Read the model definition and answer for the solid it produces. Units are mm, in the model's axes. Face numbers are marked on the shaded views. Coordinates: 2 decimals unless noted, no trailing zeros. Loops run counter-clockwise (first coordinate to the right, second up) from the corner with the lowest first, then second, coordinate; pieces in that order, holes last.
from build123d import *

# Parameters (mm, degrees)
SKETCH1_W           = 350
SKETCH1_H           = 56.2
BOSS_EXTRUDE1_DEPTH = 10
SKETCH2_W           = 56.2
SKETCH2_H           = 56.2
CUT_EXTRUDE1_DEPTH  = 5
SKETCH3_W           = 10
SKETCH3_H           = 56.2
BOSS_EXTRUDE2_DEPTH = 10
SKETCH4_W           = 10
SKETCH4_H           = 56.2
BOSS_EXTRUDE3_DEPTH = 10
CUT_EXTRUDE2_DEPTH  = 56.2
SKETCH6_W           = 10
SKETCH6_H           = 56.2
BOSS_EXTRUDE4_DEPTH = 10
SKETCH7_W           = 10
SKETCH7_H           = 56.2
BOSS_EXTRUDE5_DEPTH = 10
CUT_EXTRUDE3_DEPTH  = 56.2
SKETCH9_W           = 30
SKETCH9_H           = 30
CUT_EXTRUDE4_DEPTH  = 5
SKETCH10_R          = 3
CUT_EXTRUDE5_DEPTH  = 5
SKETCH11_W          = 2.5
SKETCH11_H          = 15
CUT_EXTRUDE6_DEPTH  = 7
SKETCH12_W          = 2.5
SKETCH12_H          = 15
CUT_EXTRUDE7_DEPTH  = 7
SKETCH13_W          = 100.7
SKETCH13_H          = 56.2
CUT_EXTRUDE9_DEPTH  = 10


with BuildPart() as part:
    # Sketch1 → Boss-Extrude1 (new body)
    with BuildSketch(Plane.XY):
        Rectangle(SKETCH1_W, SKETCH1_H)
    extrude(amount=BOSS_EXTRUDE1_DEPTH)

    # Sketch2 → Cut-Extrude1 (cut)
    with BuildSketch(Plane.XY.offset(10)):
        Rectangle(SKETCH2_W, SKETCH2_H)
    extrude(amount=-CUT_EXTRUDE1_DEPTH, mode=Mode.SUBTRACT)

    # Sketch3 → Boss-Extrude2 (add)
    with BuildSketch(Plane(origin=(175, 0, 0), x_dir=(0, 0, -1), z_dir=(1, 0, 0))):
        with Locations((-5, 0)):
            Rectangle(SKETCH3_W, SKETCH3_H)
    extrude(amount=BOSS_EXTRUDE2_DEPTH)

    # Sketch4 → Boss-Extrude3 (add)
    with BuildSketch(Plane.XY.offset(10)):
        with Locations((180, 0)):
            Rectangle(SKETCH4_W, SKETCH4_H)
    extrude(amount=BOSS_EXTRUDE3_DEPTH)

    # Sketch5 → Cut-Extrude2 (cut)
    with BuildSketch(Plane(origin=(0, 28.1, 0), x_dir=(1, 0, 0), z_dir=(0, 1, 0))):
        Polygon((175, -20), (185, -10), (185, -20), align=None)
    extrude(amount=-CUT_EXTRUDE2_DEPTH, mode=Mode.SUBTRACT)

    # Sketch6 → Boss-Extrude4 (add)
    with BuildSketch(Plane.ZY.offset(175)):
        with Locations((5, 0)):
            Rectangle(SKETCH6_W, SKETCH6_H)
    extrude(amount=BOSS_EXTRUDE4_DEPTH)

    # Sketch7 → Boss-Extrude5 (add)
    with BuildSketch(Plane.XY.offset(10)):
        with Locations((-180, 0)):
            Rectangle(SKETCH7_W, SKETCH7_H)
    extrude(amount=BOSS_EXTRUDE5_DEPTH)

    # Sketch8 → Cut-Extrude3 (cut)
    with BuildSketch(Plane(origin=(0, 28.1, 0), x_dir=(1, 0, 0), z_dir=(0, 1, 0))):
        Polygon((-175, -20), (-185, -10), (-185, -20), align=None)
    extrude(amount=-CUT_EXTRUDE3_DEPTH, mode=Mode.SUBTRACT)

    # Sketch9 → Cut-Extrude4 (cut)
    with BuildSketch(Plane.XY.offset(5)):
        Rectangle(SKETCH9_W, SKETCH9_H)
    extrude(amount=-CUT_EXTRUDE4_DEPTH, mode=Mode.SUBTRACT)

    # Sketch10 → Cut-Extrude5 (cut)
    with BuildSketch(Plane.XY.offset(5)):
        with Locations((21.55, 21.55)):
            Circle(SKETCH10_R)
        with Locations((-21.55, -21.55)):
            Circle(SKETCH10_R)
        with Locations((-21.55, 21.55)):
            Circle(SKETCH10_R)
        with Locations((21.55, -21.55)):
            Circle(SKETCH10_R)
    extrude(amount=-CUT_EXTRUDE5_DEPTH, mode=Mode.SUBTRACT)

    # Sketch11 → Cut-Extrude6 (cut)
    with BuildSketch(Plane(origin=(97.5, 0, 97.5), x_dir=(0.7071067811865478, 0, -0.7071067811865472), z_dir=(0.7071067811865472, 0, 0.7071067811865478))):
        with Locations((116.672618896, 0)):
            Rectangle(SKETCH11_W, SKETCH11_H)
    extrude(amount=-CUT_EXTRUDE6_DEPTH, mode=Mode.SUBTRACT)

    # Sketch12 → Cut-Extrude7 (cut)
    with BuildSketch(Plane(origin=(-97.5, 0, 97.5), x_dir=(0.7071067811865478, 0, 0.7071067811865472), z_dir=(-0.7071067811865472, 0, 0.7071067811865478))):
        with Locations((-116.672618896, 0)):
            Rectangle(SKETCH12_W, SKETCH12_H)
    extrude(amount=-CUT_EXTRUDE7_DEPTH, mode=Mode.SUBTRACT)

    # Sketch13 → Cut-Extrude9 (cut)
    with BuildSketch(Plane.XY.offset(10)):
        with Locations((-134.65, 0)):
            Rectangle(SKETCH13_W, SKETCH13_H)
        with Locations((134.65, 0)):
            Rectangle(SKETCH13_W, SKETCH13_H)
    extrude(amount=-CUT_EXTRUDE9_DEPTH, mode=Mode.SUBTRACT)


with BuildPart() as body_2:
    # of the pieces the cut leaves, the one that is kept (cut_extrude9_keep)
    add(part.part.solids().sort_by_distance((-84.3, -28.1, 0))[0])


solid = body_2.part
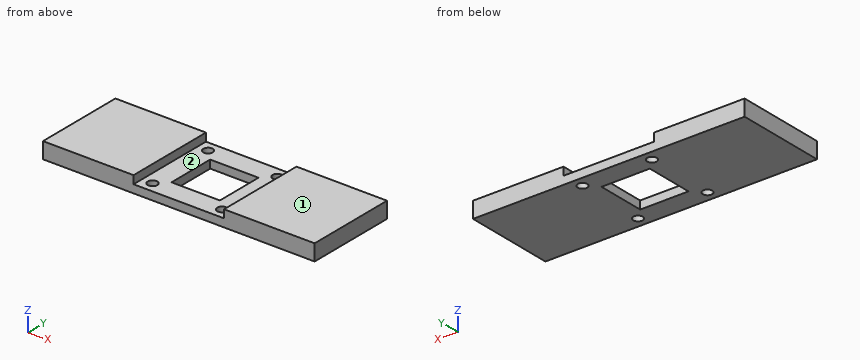
Item 1: A cutting plane is placed at A-A on z = 6.75. Determine the outline of the cut face in (x, y), then the cut area to 3 significant figures.
Numbers:
outline: (-84.3, -28.1) - (-28.1, -28.1) - (-28.1, 28.1) - (-84.3, 28.1) - close; (28.1, -28.1) - (84.3, -28.1) - (84.3, 28.1) - (28.1, 28.1) - close
area: 6,320 mm2
Item 2: A cutting plane is placed at B-B on x = -21.55. Determine the outline of the cut face in (y, z).
Numbers:
outline: (-28.1, 0) - (-24.55, 0) - (-24.55, 5) - (-28.1, 5) - close; (-18.55, 0) - (18.55, 0) - (18.55, 5) - (-18.55, 5) - close; (24.55, 0) - (28.1, 0) - (28.1, 5) - (24.55, 5) - close
Item 3: Given pin 1 (5 mm diameter, centred on x = -21.55, y = 21.55, fed in from +Z); pin 2 (9.5 mm diameter, centred on x = -21.55, y = -21.55, fed in from +Z), each flat-ended and moving along its own axis, determine where each tip first touches the part or whether it passes through.
Numbers:
pin 1: passes through
pin 2: stops at z = 5
Item 4: Determine the mould class of the marked faces 1 and 2 for opening direction X: released by +X, released by -X, zero draft, split by the parting line, or undercut.
Numbers:
face 1: zero draft
face 2: undercut
Item 5: Find the intervals of material crossed by line 1 along Y through (x, z) = (-21.55, 2.9); line 2 along X through (y, z) = (-25, 9); line 3 along Z through (x, y) = (-15.5, 12.5), in increasing order.
Numbers:
line 1: y = -28.1 to -24.55, -18.55 to 18.55, 24.55 to 28.1
line 2: x = -84.3 to -28.1, 28.1 to 84.3
line 3: z = 0 to 5
Item 6: A cutting plane is placed at C-C on y = 3.5. Determine the outline of the cut face in (x, z).
Numbers:
outline: (-84.3, 0) - (-15, 0) - (-15, 5) - (-28.1, 5) - (-28.1, 10) - (-84.3, 10) - close; (15, 0) - (84.3, 0) - (84.3, 10) - (28.1, 10) - (28.1, 5) - (15, 5) - close
Item 7: A cutting plane is placed at D-D on y = 21.55. Determine the outline of the cut face in (x, z).
Numbers:
outline: (-84.3, 0) - (-24.55, 0) - (-24.55, 5) - (-28.1, 5) - (-28.1, 10) - (-84.3, 10) - close; (-18.55, 0) - (18.55, 0) - (18.55, 5) - (-18.55, 5) - close; (24.55, 0) - (84.3, 0) - (84.3, 10) - (28.1, 10) - (28.1, 5) - (24.55, 5) - close
